Read the model definition and answer for the solid it produces. Units are mm, in the model's axes. Face numbers are marked on the shaded views. A direction names the side the tool comes from. Round coordinates to 2 decimals unless told otherwise and drop trailing zeros. Write each loop counter-clockwise with the first axis right and the second up, starting at its lowest first coordinate (ties: lowest second). Pieces come first, ordered by that corner, then holes. Notation, with made-up numbers: (-16.75, 68) - (4.25, 68) arc R28 ccw to (4.25, 97) - close; hole circle Ø9 at (17.5, 76). An arc over 180 degrees is marked (long way). Answer as CSV lines item,"result". Start each with the question number.
1) Which of the six approach directions +Z, -Z, +X, -X, +Y, -Y give full straight-line access (tool end or side, diameter ignored) to the marked faces 5 and 6?
2) Find section A-A on x = 19. Determine the outline of the cut face in (y, z), then the cut area to 3 significant figures.
3) For a pull along X with two mould halves and no side action, classify the marked faces 1, 2, 3 and 4 as +X half, -X half, draft (parallel to the pull), parting line (faces both ways), or undercut.
4) Find section B-B on x = -0.65. Determine the outline of the cut face in (y, z), then the cut area to 3 significant figures.
5) Find section C-C on z = -4.5. Determine the outline of the cut face in (x, y).
6) Each of these flat-tipped pins is pushed along its axis until it touches: pin 1 (1.5 mm diameter, centred on x = 23, y = -9.5, fed in from -Z); pin 2 (1.5 mm diameter, centred on x = -3, z = -0.5, fed in from -Y); pin 3 (2.5 mm diameter, centred on y = -7.5, z = -3, fed in from -X); pin 4 (6 mm diameter, centred on x = 22.5, y = -1, fed in from -Z). Where does it stop, or does it pass through?
7) Consider line 1 along Y through (x, z) = (-0.65, 0.3); line 2 along Y through (x, z) = (18, 0.25); line 3 along Z through (x, y) = (34.5, -10.25). Determine where each line is inside the solid, lowest interval first.
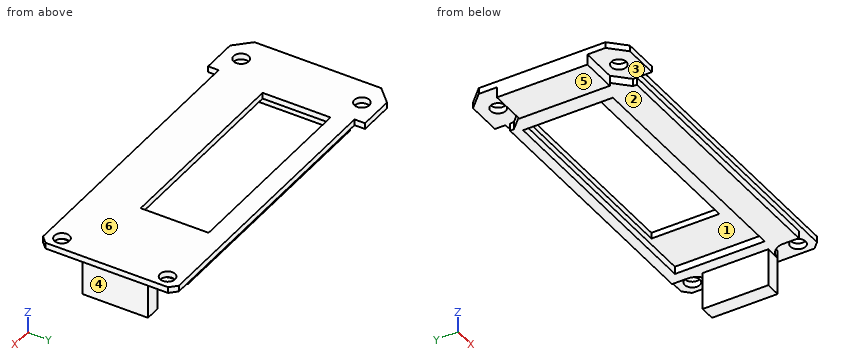
Autodesk Inventor part; units mm, degrees
ref_plane "YZ Plane" through (0, 0, 0) normal (1, 0, 0) x (0, 1, 0)
ref_plane "XZ Plane" through (0, 0, 0) normal (0, 1, 0) x (-1, 0, 0)
ref_plane "XY Plane" through (0, 0, 0) normal (0, 0, 1) x (1, 0, 0)
sketch "Эскиз1" plane through (0, 0, 0) normal (0, 0, 1) x (1, 0, 0)
  line L0 (40.25, 0.65) -> (37.25, 0.65)
  line L1 (37.25, 0.65) -> (37.25, -2.2)
  arc A0 (37.25, -2.2) -> (39.25, -4.2) centre (39.25, -2.2) ccw
  line L2 (39.25, -4.2) -> (39.25, -12.9)
  arc A1 (39.25, -12.9) -> (37.25, -14.9) centre (39.25, -14.9) ccw
  line L3 (37.25, -14.9) -> (37.25, -17.75)
  line L4 (37.25, -17.75) -> (40.25, -17.75)
  line L5 (40.25, -17.75) -> (41.25, -16.75)
  line L6 (41.25, -16.75) -> (41.25, -0.35)
  line L7 (41.25, -0.35) -> (40.25, 0.65)
  circle A2 centre (39.3375, -15.55) radius 1
  circle A3 centre (39.3375, -1.55) radius 1
  line L8 (2.55, -18.95) -> (2.55, -17.75)
  line L9 (2.55, -17.75) -> (2.55, -16.45)
  line L10 (0.65, -14.55) -> (2.55, -16.45)
  line L11 (-4.15, -14.55) -> (0.65, -14.55)
  line L12 (-4.15, -14.55) -> (-4.15, -16.95)
  line L13 (-4.15, -16.95) -> (-2.15, -18.95)
  line L14 (-2.15, -18.95) -> (2.55, -18.95)
  circle A4 centre (-0.65, -16.55) radius 1
  line L15 (2.55, 0.65) -> (2.55, 1.85)
  line L16 (2.55, 1.85) -> (-2.15, 1.85)
  line L17 (-2.15, 1.85) -> (-4.15, -0.15)
  line L18 (-4.15, -0.15) -> (-4.15, -2.55)
  line L19 (0.65, -2.55) -> (-4.15, -2.55)
  line L20 (2.55, -0.65) -> (0.65, -2.55)
  line L21 (2.55, -0.65) -> (2.55, 0.65)
  circle A5 centre (-0.65, -0.55) radius 1
  line L22 (2.55, 0.65) -> (40.25, 0.65)
  line L23 (40.25, -17.75) -> (2.55, -17.75)
  line L24 (-4.15, -14.55) -> (-4.15, -2.55)
  point P0 (0, 0)
extrude "Выдавливание1" add sketch "Эскиз1" along normal blind 0.8
sketch "Эскиз2" plane through (0, 0, 0.8) normal (0, 0, 1) x (1, 0, 0)
  line L0 (3.65, -11.05) -> (29.75, -11.05)
  line L1 (29.75, -11.05) -> (29.75, -2.05)
  line L2 (29.75, -2.05) -> (3.65, -2.05)
  line L3 (3.65, -2.05) -> (3.65, -11.05)
  line L4 (40.25, 0.65) -> (2.55, 0.65)
  line L5 (41.25, -16.75) -> (41.25, -0.35)
  point P0 (0, 0)
  dimension "d2" = 9
  dimension "d3" = 26.1
  dimension "d4" = 2.7
  dimension "d5" = 11.5
extrude "Выдавливание2" cut sketch "Эскиз2" against normal through all
sketch "Эскиз3" plane through (0, 0, 0) normal (0, 0, -1) x (-1, 0, 0)
  line L0 (-40.25, 0.65) -> (-37.25, 0.65)
  line L1 (-37.25, 0.65) -> (-37.25, -2.2)
  arc A0 (-39.25, -4.2) -> (-37.25, -2.2) centre (-39.25, -2.2) ccw
  line L2 (-39.25, -4.2) -> (-39.25, -12.9)
  arc A1 (-37.25, -14.9) -> (-39.25, -12.9) centre (-39.25, -14.9) ccw
  line L3 (-37.25, -14.9) -> (-37.25, -17.75)
  line L4 (-37.25, -17.75) -> (-40.25, -17.75)
  line L5 (-40.25, -17.75) -> (-41.25, -16.75)
  line L6 (-41.25, -16.75) -> (-41.25, -0.35)
  line L7 (-41.25, -0.35) -> (-40.25, 0.65)
  circle A2 centre (-39.3375, -15.55) radius 1
  circle A3 centre (-39.3375, -1.55) radius 1
  line L8 (-2.55, 0.65) -> (-2.55, 1.85)
  line L9 (-2.55, 1.85) -> (2.15, 1.85)
  line L10 (2.15, 1.85) -> (4.15, -0.15)
  line L11 (4.15, -0.15) -> (4.15, -2.55)
  line L12 (-0.65, -2.55) -> (4.15, -2.55)
  line L13 (-2.55, -0.65) -> (-0.65, -2.55)
  line L14 (-2.55, -0.65) -> (-2.55, 0.65)
  circle A4 centre (0.65, -0.55) radius 1
  line L15 (-2.55, -18.95) -> (-2.55, -17.75)
  line L16 (-2.55, -17.75) -> (-2.55, -16.45)
  line L17 (-0.65, -14.55) -> (-2.55, -16.45)
  line L18 (4.15, -14.55) -> (-0.65, -14.55)
  line L19 (4.15, -14.55) -> (4.15, -16.95)
  line L20 (4.15, -16.95) -> (2.15, -18.95)
  line L21 (2.15, -18.95) -> (-2.55, -18.95)
  circle A5 centre (0.65, -16.55) radius 1
  line L22 (-2.55, -17.75) -> (-40.25, -17.75)
  line L23 (4.15, -2.55) -> (4.15, -14.55)
  line L24 (4.15, -0.15) -> (4.15, -16.95)
  line L25 (-3.25, -13.35) -> (-35.75, -13.35)
  line L26 (-35.75, -13.35) -> (-35.75, -1.45)
  line L27 (-35.75, -1.45) -> (-3.25, -1.45)
  line L28 (-3.25, -1.45) -> (-3.25, -13.35)
  line L29 (-29.75, -11.05) -> (-29.75, -2.05)
  line L30 (-3.65, -11.05) -> (-29.75, -11.05)
  line L31 (-3.65, -2.05) -> (-3.65, -11.05)
  line L32 (-29.75, -2.05) -> (-3.65, -2.05)
  line L33 (2.15, 1.85) -> (-43.25, 1.85)
  line L34 (-43.25, -18.95) -> (2.15, -18.95)
  line L35 (-37.25, -0.15) -> (-2.55, -0.15)
  line L36 (-37.25, -16.95) -> (-2.55, -16.95)
  point P0 (0, 0)
  dimension "d13" = 6
  dimension "d15" = 0.4
  dimension "d17" = 2.3
  dimension "d18" = 0.6
  dimension "d21" = 2
  dimension "d22" = 2
extrude "Выдавливание3" add sketch "Эскиз3" along normal blind 1 contours L35 L14 L13 L12 L23 L18 L17 L16 L36 L3 A1 L2 A0 L1
sketch "Эскиз4" plane through (0, 0, -1) normal (0, 0, -1) x (-1, 0, 0)
  line L0 (-0.65, -2.55) -> (4.15, -2.55)
  line L1 (-2.55, -16.45) -> (-0.65, -14.55)
  line L2 (4.15, -2.55) -> (-0.65, -2.55)
  line L3 (-0.65, -2.55) -> (-0.65, -14.55)
  line L4 (-0.65, -14.55) -> (4.15, -14.55)
  line L5 (4.15, -14.55) -> (4.15, -2.55)
  point P0 (0, 0)
extrude "Выдавливание4" add sketch "Эскиз4" along normal blind 0.4
sketch "Эскиз5" plane through (0, 0, -1) normal (0, 0, -1) x (-1, 0, 0)
  line L0 (-39.25, -4.2) -> (-39.25, -12.9)
  line L1 (-39.25, -4.2) -> (-37.25, -4.2)
  line L2 (-37.25, -4.2) -> (-37.25, -12.9)
  line L3 (-37.25, -12.9) -> (-39.25, -12.9)
  line L4 (-39.25, -12.9) -> (-39.25, -4.2)
  point P0 (0, 0)
  dimension "d25" = 2
extrude "Выдавливание5" add sketch "Эскиз5" along normal blind 5
sketch "Эскиз7" plane through (0, 0, 0.8) normal (0, 0, 1) x (1, 0, 0)
  line L0 (2.55, -17.75) -> (40.25, -17.75)
  line L1 (2.55, -17.75) -> (2.55, -17.55)
  line L2 (2.55, -17.55) -> (40.1672, -17.55)
  line L3 (40.1672, -17.55) -> (41.05, -16.6672)
  line L4 (41.05, -16.6672) -> (41.05, -8.55)
  line L5 (41.25, -16.75) -> (41.25, -0.35)
  line L6 (41.25, -8.55) -> (-4.15, -8.55)
  line L7 (-4.15, -0.15) -> (-4.15, -16.95)
  line L8 (40.25, -17.75) -> (41.25, -16.75)
  line L9 (2.55, 0.45) -> (40.1672, 0.45)
  line L10 (40.1672, 0.45) -> (41.05, -0.4328)
  line L11 (41.05, -0.4328) -> (41.05, -8.55)
  line L12 (35.75, -1.45) -> (35.75, -13.35)
  line L13 (29.75, -11.05) -> (3.65, -11.05)
  line L14 (3.65, -11.05) -> (3.65, -2.05)
  line L15 (3.65, -2.05) -> (29.75, -2.05)
  line L16 (29.75, -2.05) -> (29.75, -11.05)
  line L17 (-4.15, -0.15) -> (-4.15, -16.95)
  line L18 (-4.15, -16.95) -> (-2.15, -18.95)
  line L19 (-2.15, -18.95) -> (2.55, -18.95)
  line L20 (2.55, -18.95) -> (2.55, -17.75)
  line L21 (2.55, -17.75) -> (40.25, -17.75)
  line L22 (40.25, -17.75) -> (41.25, -16.75)
  line L23 (41.25, -16.75) -> (41.25, -0.35)
  line L24 (41.25, -0.35) -> (40.25, 0.65)
  line L25 (40.25, 0.65) -> (2.55, 0.65)
  line L26 (2.55, 0.65) -> (2.55, 1.85)
  line L27 (2.55, 1.85) -> (-2.15, 1.85)
  line L28 (-2.15, 1.85) -> (-4.15, -0.15)
  circle A0 centre (-0.65, -16.55) radius 1
  circle A1 centre (-0.65, -0.55) radius 1
  circle A2 centre (39.3375, -1.55) radius 1
  circle A3 centre (39.3375, -15.55) radius 1
  line L29 (2.55, 0.45) -> (2.55, 0.65)
  line L30 (40.25, 0.65) -> (2.55, 0.65)
  line L31 (2.55, 0.65) -> (40.25, 0.65)
  line L32 (41.25, -0.35) -> (40.25, 0.65)
  line L33 (40.25, 0.65) -> (41.25, -0.35)
  point P0 (0, 0)
  dimension "d33" = 0.2
  dimension "d34" = 0.2
  dimension "d35" = 0.2
extrude "Выдавливание7" cut sketch "Эскиз7" against normal through all contours L1 L2 L3 L4 L6 L5 L8 L0 | L6 L11 L10 L9 L29 L25 L24 L5
Check values:
1,face 5,"-Z, -X, +Y, -Y"
1,face 6,"+Z, +X, -X, +Y, -Y"
2,outline,"(-17.55, 0) - (-16.95, 0) - (-16.95, -1) - (-13.35, -1) - (-13.35, 0) - (-11.05, 0) - (-11.05, 0.8) - (-17.55, 0.8) - close; (-2.05, 0) - (-1.45, 0) - (-1.45, -1) - (-0.15, -1) - (-0.15, 0) - (0.45, 0) - (0.45, 0.8) - (-2.05, 0.8) - close"
2,area,"12.1 mm^2"
3,face 1,"undercut"
3,face 2,"undercut"
3,face 3,"draft"
3,face 4,"+X half"
4,outline,"(-18.95, 0) - (-17.55, 0) - (-17.55, 0.8) - (-18.95, 0.8) - close; (-15.55, 0) - (-14.55, 0) - (-14.55, -1.4) - (-2.55, -1.4) - (-2.55, 0) - (-1.55, 0) - (-1.55, 0.8) - (-15.55, 0.8) - close; (0.45, 0) - (1.85, 0) - (1.85, 0.8) - (0.45, 0.8) - close"
4,area,"30.2 mm^2"
5,outline,"(37.25, -12.9) - (39.25, -12.9) - (39.25, -4.2) - (37.25, -4.2) - close"
6,pin 1,"passes through"
6,pin 2,"stops at y = -18.66"
6,pin 3,"stops at x = 37.25"
6,pin 4,"stops at z = -1"
7,line 1,"y = -18.95 to -17.55, -15.55 to -1.55, 0.45 to 1.85"
7,line 2,"y = -17.55 to -11.05, -2.05 to 0.45"
7,line 3,"z = 0 to 0.8"
